```python
from build123d import *

# Parameters (mm, degrees)
SKETCH1_R           = 11.811
BOSS_EXTRUDE1_DEPTH = 10
BOSS_EXTRUDE2_START = -10
BOSS_EXTRUDE2_DEPTH = 10
CIRPATTERN1_COUNT   = 18


with BuildPart() as part:
    # Sketch1 → Boss-Extrude1 (new body)
    with BuildSketch(Plane(origin=(0, 0, 0), x_dir=(1, 0, 0), z_dir=(0, 1, 0))):
        with Locations(Location((0, 0, 0), (0, 0, 270))):
            Circle(SKETCH1_R)
        Polygon((0, 5.600297611), (-4.85, 2.800148806), (-4.85, -2.800148806), (0, -5.600297611), (4.85, -2.800148806), (4.85, 2.800148806), align=None, mode=Mode.SUBTRACT)
    extrude(amount=BOSS_EXTRUDE1_DEPTH)

    # Sketch2 → Boss-Extrude2 (add)
    with BuildSketch(Plane(origin=(0, 10, 0), x_dir=(1, 0, 0), z_dir=(0, 1, 0)).offset(BOSS_EXTRUDE2_START)):
        with BuildLine():
            ThreePointArc((0.889, 12.7), (0, 13.589), (-0.889, 12.7))
            ThreePointArc((-0.889, 12.7), (-1.070430373, 12.103223599), (-1.553320634, 11.70841219))
            ThreePointArc((-1.553320634, 11.70841219), (0, 11.811), (1.553320634, 11.70841219))
            ThreePointArc((1.553320634, 11.70841219), (1.070430373, 12.103223599), (0.889, 12.7))
        make_face()
    boss_extrude2 = extrude(amount=BOSS_EXTRUDE2_DEPTH)

    # CirPattern1: Boss-Extrude2 ×18 about axis
    cirpattern1_axis = Axis((0, 0, 0), (0, 1, 0))
    for i in range(1, CIRPATTERN1_COUNT):
        add(boss_extrude2.rotate(cirpattern1_axis, i * 360 / CIRPATTERN1_COUNT))


solid = part.part
```
Build history of the part. All positions in model axes, mm. A direction names the side the tool comes from. Round coordinates to 2 decimals unless told otherwise and drop trailing zeros. Loops run counter-clockwise (first coordinate to the right, second up) from the corner with the lowest first, then second, coordinate; pieces in that order, holes last.
Item 1: Which spindle directions (+Z, -Z, +X, -X, +Y, -Y) get a long thin tool onto all of the face, cutting with end or side? Do faces 4 (the face through (-11.101, 4.93, 4.033)), 5 (the face through (-2.46, 4.93, 4.18)), 6 (the face through (11.101, 4.93, -4.033)), 7 (the face through (-2.044, 4.93, -11.633)). Say none if no direction does.
Item 2: Drill centre lines: line 1 along X through (y, z) = (5.5, 0.25); line 2 along X through (y, z) = (5.75, 5); line 3 along Z through (x, y) = (8.5, 4.5). Where is each one in solid material? Low to high.
Item 3: Pin check, flat tips, straight feed: P1, Ø1.5, axis at x = -10, y = 8, coming from the -Z side; P2, Ø1, axis at x = -2.5, y = 5.5, coming from the -Z side; P3, Ø1, axis at x = 5, y = 9, coming from the +Z side. Stop position of each tip, or through.
Item 4: Saw through at A-A (z = 6.35). List the corners of the cut face in (x, y).
Item 5: Two-plate mould, pull along Z, no slides. Class faces 1 (the face through (-5.912, 4.93, 10.225)), 2 (the face through (13.386, 4.93, -2.34)), 3 (the face through (-5.9, 4.93, -10.23)): released by +Z, released by -Z, zero draft, split by the parting line, or undercut.
Worked answers:
1. face 4: -X, +Y, -Y
1. face 5: +Y, -Y
1. face 6: +X, +Y, -Y
1. face 7: -Z, +Y, -Y
2. line 1: x = -11.81 to -4.85, 4.85 to 11.81
2. line 2: x = -10.97 to -1.04, 1.04 to 10.97
2. line 3: z = -10.55 to 10.55
3. P1: stops at z = -7.34
3. P2: stops at z = -11.66
3. P3: stops at z = 12.81
4. outline: (-11.89, 0) - (11.89, 0) - (11.89, 10) - (-11.89, 10) - close
5. face 1: released by +Z
5. face 2: undercut
5. face 3: released by -Z
